Geometry check sheet. Reference: the model listing, model coordinates, mm. Face numbers are marked on the shaded views. A direction names the side the tool comes from. Round coordinates to 2 decimals unless told otherwise and drop trailing zeros. Write each loop counter-clockwise with the first axis right and the second up, starting at its lowest first coordinate (ties: lowest second). Pieces come first, ordered by that corner, then holes. Notation, with made-up numbers: (1, 86.25) - (16, 86.25) arc R19 cw to (16, 102.25) - close; hole circle Ø4 at (50, 77.25). An arc over 180 degrees is marked (long way). Return JSON: item names as keys, results as strings.
```python
from build123d import *

# Parameters (mm, degrees)
PAD_DEPTH     = 20
POCKET_DEPTH  = 10.001
CHAMFER_SIZE2 = 3.5
CHAMFER_SIZE  = 2
FILLET_R      = 2


with BuildPart() as part:
    # Sketch → Pad (new body)
    with BuildSketch(Plane.XZ):
        Polygon((0, 0), (27, 0), (26, 10), (1, 10), align=None)
    extrude(amount=PAD_DEPTH)

    # Sketch001 (on Face1 of Pad) → Pocket (cut, through all)
    with BuildSketch(Plane(origin=(0, 0, 0), x_dir=(1, 0, 0), z_dir=(0, 0, -1))):
        with BuildLine():
            ThreePointArc((12.5, 12.25), (10.25, 10), (12.5, 7.75))
            Line((12.5, 7.75), (14.5, 7.75))
            ThreePointArc((14.5, 7.75), (16.75, 10), (14.5, 12.25))
            Line((12.5, 12.25), (14.5, 12.25))
        make_face()
    extrude(amount=-POCKET_DEPTH, mode=Mode.SUBTRACT)

    # Chamfer
    chamfer_edges = [part.edges().sort_by_distance(p)[0] for p in [
        (10.25, -10, 0),
        (13.5, -12.25, 0),
        (16.75, -10, 0),
        (13.5, -7.75, 0),
    ]]
    chamfer_side = part.faces().sort_by_distance((0.336006, -10, 0))[0]
    chamfer(chamfer_edges, length=CHAMFER_SIZE, length2=CHAMFER_SIZE2, reference=chamfer_side)

    # Fillet
    fillet_edges = [part.edges().sort_by_distance(p)[0] for p in [
        (26.5, -20, 5),
        (0.5, -20, 5),
        (26.5, 0, 5),
        (0.5, 0, 5),
    ]]
    fillet(fillet_edges, radius=FILLET_R)


solid = part.part
```
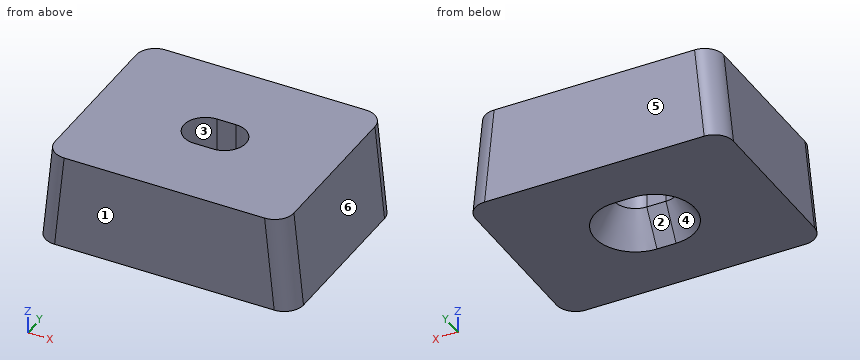
(1) Section check B-B, the plane y = -15. Enter the section's corners in (x, z), plus the area to 3 significant figures.
Response values:
{"outline": "(0, 0) - (27, 0) - (26, 10) - (1, 10) - close", "area": "260 mm^2"}
(2) Section check C-C, the plane y = -1.5. Enter the section's corners in (x, z), plus the area to 3 significant figures.
Response values:
{"outline": "(0.06, 0) - (26.94, 0) - (25.94, 10) - (1.06, 10) - close", "area": "259 mm^2"}
(3) Section check A-A, the plane y = -10. Enter the section's corners in (x, z).
Response values:
{"outline": "(0, 0) - (8.25, 0) - (10.25, 3.5) - (10.25, 10) - (1, 10) - close; (16.75, 3.5) - (18.75, 0) - (27, 0) - (26, 10) - (16.75, 10) - close"}
(4) Gauge pin test, flat ends, axial feed: pin 1 (3 mm diameter, centred on x = 11, y = -9.5, fed in from +Z); pin 2 (3 mm diameter, centred on y = -13.5, z = 4, fed in from -X); pin 3 (4 mm diameter, centred on y = -16.5, z = 7.5, fed in from -X). Record the tip position at first contact, or that the pin passes through.
Response values:
{"pin 1": "stops at z = 10", "pin 2": "stops at x = 0.25", "pin 3": "stops at x = 0.55"}
(5) Material ranges on line 1 along X through (y, z) = (-11.5, 8.25) (3 decimals); line 2 along Y through (x, z) = (12.75, 8.5); line 3 along Y through (x, z) = (15.5, 1.25), recorded low to high. Write a range as [from, to].
Response values:
{"line 1": "x = [0.825, 10.823], [16.177, 26.175]", "line 2": "y = [-20, -12.25], [-7.75, 0]", "line 3": "y = [-20, -13.39], [-6.61, 0]"}
(6) Access from +Z, -Z, +X, -X, +Y, -Y to the whole of each face (thin tool, end or side, straight path). Record for the marked faces 1, 2 and 3.
Response values:
{"face 1": "+Z, -Z, +X, -X, -Y", "face 2": "-Z", "face 3": "+Z, -Z"}
(7) Release check for a two-part mould opening along X. For the marked faces 4, 5 and 6 record: pulls with the +X half, pulls with the -X half, needs draft (parallel to the pull), parting line crosses it, or undercut.
Response values:
{"face 4": "undercut", "face 5": "needs draft", "face 6": "pulls with the +X half"}
